Check sheet for the modelled part. Datum: model origin and axes. Units: mm. A direction names the side the tool comes from. Coordinates: 2 decimals unless noted, no trailing zeros. Loops run counter-clockwise (first coordinate to the right, second up) from the corner with the lowest first, then second, coordinate; pieces in that order, holes last. Notation, with made-up numbers: M 76,72 L 85,72 A31 cw 85,104 Z; hole C 71.5,34.5 d7. An arc over 180 degrees is marked long. Use CSV: the item, a comma, the result in double quotes. Start each with the question number.
(1) Section check B-B on y = -29.5. Record the cut outline in (x, z), and give its area (4 significant figures).
(2) Go/stop test with flat-tipped pins: pin 1 Ø11 at (y, z) = (16, 9.5) entering from +X; pin 2 Ø1.6 at (x, z) = (59, 0.5) entering from +Y; pin 3 Ø8 at (y, z) = (3.5, 18.5) entering from -X. Record where each tip stops, or that it passes through.
(3) Scan lines: line 1 (Y direction, x = -31.5, z = 13); line 2 (X direction, y = 14, z = 7); line 3 (Z direction, x = -57, y = 0). Record each from-to range of solid material in increasing order.
(4) Set-up check for faces 5 (the flat face through (-1, 0, 0)), 6 (the flat face through (1, -32.5, 8)): record each of +Z, -Z, +X, -X, +Y, -Y from which the full face is reachable in a straight line by a thin tool's end or side.
(5) Section check C-C on x = -24. Record the cut outline in (y, z).
(6) Section check A-A on z = 12.25. Record the cut outline in (x, y).
(7) Draft check along X on faces 1 (the cylindrical face through (-66.04, -3.777, 0.76)), 2 (the flat face through (-0.3, 33.5, 14.5)), 3 (the flat face through (-1, 32.5, 8)), 4 (the cylindrical face through (66.04, 3.777, 0.76)). Enter one of: pulls with the +X half, pulls with the -X half, needs draft (parallel to the pull), parting line crosses it, or undercut.
from build123d import *

# Parameters (mm, degrees)
F1_DEPTH  = 1.5
F3_DEPTH  = 13
F4_R      = 2.003864
F5_DEPTH  = 2
F6_R      = 5
F7_W      = 1.5
F7_H      = 10.848721
F8_DEPTH  = 8
F9_R      = 4
F10_R     = 2.560251
F11_DEPTH = 125


with BuildPart() as f1:
    # F0 (on Top) → F1 (new body)
    with BuildSketch(Plane.XY):
        Polygon((57.5, 5.202384), (57.5, 34), (-57.5, 34), (-57.5, 5.202384), (-57.5, -5.202384), (-57.5, -34), (57.5, -34), (57.5, -5.202384), (57.5, 0), align=None)
        Polygon((-57.5, -5.202384), (-57.5, 5.202384), (-67.543589, 5.202384), (-67.543589, 0), (-67.543589, -5.202384), align=None)
        Polygon((67.543589, 5.202384), (57.5, 5.202384), (57.5, 0), (57.5, -5.202384), (67.543589, -5.202384), (67.543589, 0), align=None)
    extrude(amount=F1_DEPTH)

    # F2 (on face) → F3 (join)
    with BuildSketch(Plane.XY.offset(1.5)):
        Polygon((-57.5, 34), (-57.5, 5.202384), (-57.5, -5.202384), (-57.5, -34), (57.5, -34), (57.5, -5.202384), (57.5, 5.202384), (57.5, 34), align=None)
        Polygon((-56, 32.5), (56, 32.5), (56, 5.202384), (56, -5.202384), (56, -32.5), (-56, -32.5), (-56, -5.202384), (-56, 5.202384), align=None, mode=Mode.SUBTRACT)
    extrude(amount=F3_DEPTH)

    # F4 (on face) → F5 (cut)
    with BuildSketch(Plane.XY.offset(1.5)):
        with Locations((-62.578715, 0)):
            Circle(F4_R)
        with Locations((62.578715, 0)):
            Circle(F4_R)
    extrude(amount=-F5_DEPTH, mode=Mode.SUBTRACT)

    # F6
    f6_edges = [f1.edges().sort_by_distance(p)[0] for p in [
        (-67.543589, 5.202384, 0.75),
        (-67.543589, -5.202384, 0.75),
        (67.543589, 5.202384, 0.75),
        (67.543589, -5.202384, 0.75),
    ]]
    fillet(f6_edges, radius=F6_R)

    # F7 (on face) → F8 (join)
    with BuildSketch(Plane.XY.offset(14.5)):
        with Locations((-56.75, -0.06754)):
            Rectangle(F7_W, F7_H)
        with Locations((56.75, -0.06754)):
            Rectangle(F7_W, F7_H)
    extrude(amount=F8_DEPTH)

    # F9
    f9_edges = [f1.edges().sort_by_distance(p)[0] for p in [
        (-56.75, -5.491901, 22.5),
        (-56.75, 5.35682, 22.5),
        (56.75, -5.491901, 22.5),
        (56.75, 5.35682, 22.5),
    ]]
    fillet(f9_edges, radius=F9_R)

    # F10 (on face) → F11 (cut)
    with BuildSketch(Plane.YZ.offset(57.5)):
        with Locations((0, 17.783318)):
            Circle(F10_R)
    extrude(amount=-F11_DEPTH, mode=Mode.SUBTRACT)


solid = f1.part
Outcome:
1,outline,"M -57.5,0 L 57.5,0 L 57.5,14.5 L 56,14.5 L 56,1.5 L -56,1.5 L -56,14.5 L -57.5,14.5 Z"
1,area,"211.5 mm²"
2,pin 1,"stops at x = 57.5"
2,pin 2,"stops at y = 5.2"
2,pin 3,"stops at x = -57.5"
3,line 1,"y = -34 to -32.5, 32.5 to 34"
3,line 2,"x = -57.5 to -56, 56 to 57.5"
3,line 3,"z = 0 to 15.22, 20.34 to 22.5"
4,face 5,"-Z, +X, -X, +Y, -Y"
4,face 6,"+Z"
5,outline,"M -34,0 L 34,0 L 34,14.5 L 32.5,14.5 L 32.5,1.5 L -32.5,1.5 L -32.5,14.5 L -34,14.5 Z"
6,outline,"M -57.5,-34 L 57.5,-34 L 57.5,34 L -57.5,34 Z; hole M -56,-32.5 L 56,-32.5 L 56,32.5 L -56,32.5 Z"
7,face 1,"pulls with the -X half"
7,face 2,"needs draft"
7,face 3,"undercut"
7,face 4,"pulls with the +X half"
